Input: part model. Units: mm. Frame: model coordinates. A direction names the side the tool comes from. Round coordinates to 2 decimals unless told otherwise and drop trailing zeros. Order: outer loops, then holes, each group sorted by start corner. A loop starts at its lowest first (then second) coordinate and runs counter-clockwise, first axis right, second up.
Item 1: Cut plane B-B on y = 63. Output: boundary loops of the cut face in (x, z) (3 decimals), then the cut area to 3 significant figures.
Item 2: Cut plane C-C on z = 2.5. Output: boundary loops of the cut face in (x, y), then the cut area to 3 significant figures.
Item 3: Cut plane A-A on x = 3. Output: boundary loops of the cut face in (y, z), then the cut area to 3 significant figures.
Item 4: Cut plane D-D on x = -2.5. Output: boundary loops of the cut face in (y, z).
Item 5: Reachability of faces 4 (the flat face through (-15.875, 34, 1)), 5 (the cylindrical face through (-3.9, -9.09, 6.84)), 6 (the flat face through (8.636, 36, 1)), 7 (the flat face through (-7.239, 35, 4)), 8 (the cylindrical face through (-3.34, 78.94, 6.84)) from +Z, -Z, +X, -X, +Y, -Y: full face, straight path, thin tool, end or side. Return the list, or none.
Item 6: Line query: L1, parallel to Z at x = -8, y = 1; L2, parallel to X at y = 15, z = 5; L3, parallel to Y at x = -3.75, z = 1.75. Output: solid intervals per line, ascending.
Item 7: First-contact query: pin 1 (0.5 mm diameter, centred on y = 26, z = 1, fed in from -X) (3 decimals); pin 2 (1 mm diameter, centred on x = -11.5, z = 3.5, fed in from -Y); pin 3 (1.5 mm diameter, centred on y = 25, z = 2.5, fed in from -X); pin 4 (2 mm diameter, centred on y = 33.5, z = 4.5, fed in from +X). Flat tips, straight axial feed; report the tip coordinate or a pass-through.
Item 8: Mould query, pull axis Z, two halves, no side actions, for faces 1 (the flat face through (-4, 36, 7.62)), 2 (the flat face through (-9, 36, 6.045)), 3 (the flat face through (-4, 34, 0)). Classes: released by +Z, released by -Z, zero draft, split by the parting line, or undercut.
```python
from build123d import *

# Parameters (mm, degrees)
F1_DEPTH = 7.62
F3_DEPTH = 1.5748
F5_DEPTH = 1.5748


with BuildPart() as f1:
    # F0 (on Top) → F1 (new body)
    with BuildSketch(Plane.XY):
        with BuildLine():
            ThreePointArc((-3.6195, 0), (-1.060127, 1.060127), (0, 3.6195))
            Line((0, 3.6195), (0, 66.2305))
            ThreePointArc((0, 66.2305), (-1.060127, 68.789873), (-3.6195, 69.85))
            ThreePointArc((-3.6195, 69.85), (-6.178873, 68.789873), (-7.239, 66.2305))
            Line((-7.239, 66.2305), (-7.239, 3.6195))
            ThreePointArc((-7.239, 3.6195), (-6.178873, 1.060127), (-3.6195, 0))
        make_face()
    extrude(amount=F1_DEPTH)

    # F2 (on face) → F3 (join)
    with BuildSketch(Plane(origin=(0, 0, 0), x_dir=(1, 0, 0), z_dir=(0, 0, -1))):
        Polygon((8.636, 11.456368), (-3.6195, 15.813879), (-15.875, 11.456368), (-15.875, -3.6195), (-15.875, -66.2305), (-15.875, -81.306368), (-3.6195, -85.663879), (8.636, -81.306368), (8.636, -66.2305), (8.636, -3.6195), align=None)
        with BuildLine():
            ThreePointArc((-7.239, -3.6195), (-3.6195, 0), (0, -3.6195))
            Line((0, -3.6195), (0, -66.2305))
            ThreePointArc((0, -66.2305), (-3.6195, -69.85), (-7.239, -66.2305))
            Line((-7.239, -66.2305), (-7.239, -3.6195))
        make_face(mode=Mode.SUBTRACT)
    extrude(amount=-F3_DEPTH)

    # F4 (on face) → F5 (join)
    with BuildSketch(Plane.XY.offset(7.62)):
        with BuildLine():
            ThreePointArc((9.0932, 66.2305), (-3.6195, 78.9432), (-16.3322, 66.2305))
            Line((-16.3322, 66.2305), (-16.3322, 3.6195))
            ThreePointArc((-16.3322, 3.6195), (-3.6195, -9.0932), (9.0932, 3.6195))
            Line((9.0932, 3.6195), (9.0932, 66.2305))
        make_face()
        with BuildLine():
            ThreePointArc((0, 3.6195), (-3.6195, 0), (-7.239, 3.6195))
            Line((-7.239, 3.6195), (-7.239, 66.2305))
            ThreePointArc((-7.239, 66.2305), (-3.6195, 69.85), (0, 66.2305))
            Line((0, 66.2305), (0, 3.6195))
        make_face(mode=Mode.SUBTRACT)
    extrude(amount=-F5_DEPTH)


solid = f1.part
```
From the geometry:
1. outline: (-16.332, 6.045) - (-7.239, 6.045) - (-7.239, 1.575) - (-15.875, 1.575) - (-15.875, 0) - (8.636, 0) - (8.636, 1.575) - (0, 1.575) - (0, 6.045) - (9.093, 6.045) - (9.093, 7.62) - (-16.332, 7.62) - close
1. area: 111 mm2
2. outline: (-7.24, 3.62) arc R3.62 ccw to (0, 3.62) - (0, 66.23) arc R3.62 ccw to (-7.24, 66.23) - close
2. area: 494 mm2
3. outline: (-13.46, 0) - (83.31, 0) - (83.31, 1.57) - (-13.46, 1.57) - close; (-7.23, 6.05) - (77.08, 6.05) - (77.08, 7.62) - (-7.23, 7.62) - close
3. area: 285 mm2
4. outline: (-15.42, 0) - (85.27, 0) - (85.27, 1.57) - (69.67, 1.57) - (69.67, 6.05) - (78.89, 6.05) - (78.89, 7.62) - (-9.04, 7.62) - (-9.04, 6.05) - (0.18, 6.05) - (0.18, 1.57) - (-15.42, 1.57) - close
5. face 4: -Z, -X, +Y, -Y
5. face 5: +Z, -Y
5. face 6: -Z, +X, +Y, -Y
5. face 7: -X, +Y, -Y
5. face 8: +Z, +Y
6. L1: z = 0 to 1.57, 6.05 to 7.62
6. L2: x = -7.24 to 0
6. L3: y = 0 to 69.85
7. pin 1: stops at x = -15.875
7. pin 2: passes through
7. pin 3: stops at x = -7.24
7. pin 4: stops at x = 0
8. face 1: released by +Z
8. face 2: undercut
8. face 3: released by -Z
